```python
from build123d import *

# Parameters (mm, degrees)
SKETCH2_W                = 26
SKETCH2_H                = 25
BOSS_EXTRUDE1_DEPTH      = 0.8
SKETCH3_R                = 3.85
CUT_EXTRUDE1_DEPTH       = 19.05242366
BOSS_EXTRUDE2_DEPTH      = 8.2
BOSS_EXTRUDE2_DEPTH_BACK = 0.8
SKETCH4_W                = 30
SKETCH4_H                = 29
SKETCH4_W_2              = 26
SKETCH4_H_2              = 25
SKETCH5_W                = 30
SKETCH5_H                = 29
SKETCH5_W_2              = 25
SKETCH5_H_2              = 24
BOSS_EXTRUDE3_DEPTH      = 0.8
SKETCH6_W                = 30
SKETCH6_H                = 29
SKETCH6_W_2              = 28
SKETCH6_H_2              = 27.066666666
BOSS_EXTRUDE4_DEPTH      = 1
BOSS_EXTRUDE5_DEPTH      = 4.55
SKETCH8_W                = 17
SKETCH8_H                = 3.928450078
CUT_EXTRUDE2_DEPTH       = 4.45
SKETCH9_W                = 4.03686976
SKETCH9_H                = 12.262943987
CUT_EXTRUDE3_DEPTH       = 4.55


with BuildPart() as part:
    # Sketch2 → Boss-Extrude1 (new body)
    with BuildSketch(Plane(origin=(0, 0, 0), x_dir=(1, 0, 0), z_dir=(0, 1, 0))):
        Rectangle(SKETCH2_W, SKETCH2_H)
    extrude(amount=BOSS_EXTRUDE1_DEPTH)

    # Sketch3 → Cut-Extrude1 (cut, through all)
    with BuildSketch(Plane(origin=(0, 0.8, 0), x_dir=(1, 0, 0), z_dir=(0, 1, 0))):
        with Locations(Location((0, -2.2, 0), (0, 0, 270))):
            Circle(SKETCH3_R)
    extrude(amount=-CUT_EXTRUDE1_DEPTH, mode=Mode.SUBTRACT)

    # Sketch4 → Boss-Extrude2 (add, two sides: drawn at the far end of the back side and taken through both)
    with BuildSketch(Plane.XZ.offset(-BOSS_EXTRUDE2_DEPTH_BACK)):
        Rectangle(SKETCH4_W, SKETCH4_H)
        Rectangle(SKETCH4_W_2, SKETCH4_H_2, mode=Mode.SUBTRACT)
    extrude(amount=BOSS_EXTRUDE2_DEPTH + BOSS_EXTRUDE2_DEPTH_BACK)

    # Sketch5 → Boss-Extrude3 (add)
    with BuildSketch(Plane.XZ.offset(8.2)):
        Rectangle(SKETCH5_W, SKETCH5_H)
        Rectangle(SKETCH5_W_2, SKETCH5_H_2, mode=Mode.SUBTRACT)
    extrude(amount=BOSS_EXTRUDE3_DEPTH)

    # Sketch6 → Boss-Extrude4 (add)
    with BuildSketch(Plane.XZ.offset(9)):
        Rectangle(SKETCH6_W, SKETCH6_H)
        Rectangle(SKETCH6_W_2, SKETCH6_H_2, mode=Mode.SUBTRACT)
    extrude(amount=BOSS_EXTRUDE4_DEPTH)

    # Sketch7 → Boss-Extrude5 (add)
    with BuildSketch(Plane.XZ):
        Polygon((-10.396843815, 11.329893901), (10.396843815, 11.329893901), (10.396843815, 7.826195619), (10.396843815, -10.644387716), (6.359974055, -10.644387716), (6.359974055, 7.826195619), (-6.359974055, 7.826195619), (-6.359974055, -10.644387716), (-10.396843815, -10.644387716), (-10.396843815, 7.826195619), align=None)
    extrude(amount=BOSS_EXTRUDE5_DEPTH)

    # Sketch8 → Cut-Extrude2 (cut)
    with BuildSketch(Plane.XZ.offset(10)):
        with Locations((0, 12.535774961)):
            Rectangle(SKETCH8_W, SKETCH8_H)
    extrude(amount=-CUT_EXTRUDE2_DEPTH, mode=Mode.SUBTRACT)

    # Sketch9 → Cut-Extrude3 (cut)
    with BuildSketch(Plane.XZ.offset(4.55)):
        with Locations((-8.378408935, -0.399878609)):
            Rectangle(SKETCH9_W, SKETCH9_H)
        with Locations((8.378408935, -0.399878609)):
            Rectangle(SKETCH9_W, SKETCH9_H)
    extrude(amount=-CUT_EXTRUDE3_DEPTH, mode=Mode.SUBTRACT)


solid = part.part
```
Geometry check sheet. Reference: the model listing, model coordinates, mm. A direction names the side the tool comes from. Coordinates: 2 decimals unless noted, no trailing zeros. Write each loop counter-clockwise with the first axis right and the second up, starting at its lowest first coordinate (ties: lowest second). Pieces come first, ordered by that corner, then holes. Notation, with made-up numbers: M -28,79.5 L 4,79.5 A14 ccw 4,85.5 Z; hole C 62.25,-24.5 d2. An arc over 180 degrees is marked long. One line per item, written item: value. Start each with the question number.
(1) Sectioned sample at C-C, the plane x = 0. Enter the section's corners in (y, z).
(2) Sectioned sample at B-B, the plane z = 2.2. Enter the section's corners in (x, y).
(3) Depth check by flat-ended pin: pin 1 (4.5 mm diameter, centred on x = 9.5, z = -8, fed in from -Y); pin 2 (2 mm diameter, centred on x = -2.5, z = -7.5, fed in from -Y). Enter the tip coordinate at first touch or a pass-through.
(4) Scan lines: line 1 along Z through (x, y) = (8.75, -1.25); line 2 along Z through (x, y) = (5.5, -2.5); line 3 along Z through (x, y) = (5, -5.25). Record each from-to range of solid material in increasing order. Write a range as [from, to].
(5) Sectioned sample at D-D, the plane z = 9. Enter the section's corners in (x, y), and give its area (3 significant figures).
(6) Tool access check on faces 1 (the face through (13, -4, 0)), 2 (the face through (-8.5, -8, 14)), 3 (the face through (11.2, -9.5, 13.533)). Record the directions out of +Z, -Z, +X, -X, +Y, -Y that give a thin tool (end or side, any length) a straight path to the whole face; none if there is none.
(7) Sectioned sample at A-A, the plane y = -3. Enter the section's corners in (x, z), and give its area (3 significant figures).
Filled sheet:
1. outline: M -10,-14.5 L 0.8,-14.5 L 0.8,-1.65 L 0,-1.65 L 0,-12.5 L -8.2,-12.5 L -8.2,-12 L -9,-12 L -9,-13.53 L -10,-13.53 Z; M -5.55,12.5 L 0,12.5 L 0,11.33 L -4.55,11.33 L -4.55,7.83 L 0,7.83 L 0,6.05 L 0.8,6.05 L 0.8,14.5 L -5.55,14.5 Z
2. outline: M -15,-10 L -14,-10 L -14,-9 L -12.5,-9 L -12.5,-8.2 L -13,-8.2 L -13,0 L -3.85,0 L -3.85,0.8 L -15,0.8 Z; M 3.85,0 L 13,0 L 13,-8.2 L 12.5,-8.2 L 12.5,-9 L 14,-9 L 14,-10 L 15,-10 L 15,0.8 L 3.85,0.8 Z
3. pin 1: y = -4.55
3. pin 2: y = 0
4. line 1: [-14.5, -12.5], [-10.64, -6.53], [5.73, 11.33], [12.5, 14.5]
4. line 2: [-14.5, -12.5], [7.83, 11.33], [12.5, 14.5]
4. line 3: [-14.5, -12.5], [12.5, 14.5]
5. outline: M -15,-10 L -14,-10 L -14,-9 L -12.5,-9 L -12.5,-8.2 L -13,-8.2 L -13,0 L -10.4,0 L -10.4,-4.55 L 10.4,-4.55 L 10.4,0 L 13,0 L 13,-8.2 L 12.5,-8.2 L 12.5,-9 L 14,-9 L 14,-10 L 15,-10 L 15,0.8 L -15,0.8 Z
5. area: 157 mm²
6. face 1: none
6. face 2: +Z, -Y
6. face 3: -Y
7. outline: M -15,-14.5 L 15,-14.5 L 15,14.5 L -15,14.5 Z; M -10.4,-10.64 L -6.36,-10.64 L -6.36,-6.53 L -10.4,-6.53 Z; M -10.4,5.73 L -6.36,5.73 L -6.36,7.83 L 6.36,7.83 L 6.36,5.73 L 10.4,5.73 L 10.4,11.33 L -10.4,11.33 Z; M 6.36,-10.64 L 10.4,-10.64 L 10.4,-6.53 L 6.36,-6.53 Z; hole M -13,-12.5 L 13,-12.5 L 13,12.5 L -13,12.5 Z
7. area: 343 mm²
